Design review of the part built by this model. Coordinates are the model's own, in mm. Face numbers are marked on the shaded views. A direction names the side the tool comes from. Give positions to 0.01 mm unless a question says otherwise; leave off trailing zeros. Order: outer loops, then holes, each group sorted by start corner. A loop starts at its lowest first (then second) coordinate and runs counter-clockwise, first axis right, second up. Notation, with made-up numbers: M 80.25,77.5 L 134.25,77.5 A35 ccw 134.25,112.5 Z; hole C -29,66 d9. An arc over 180 degrees is marked long. Answer as a JSON object with one key per item and string values.
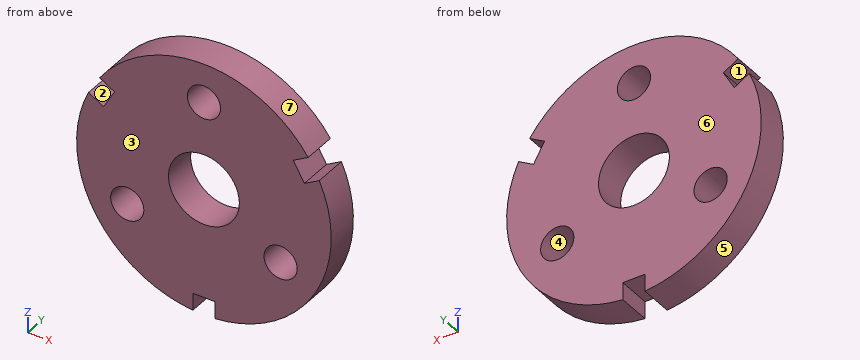
from build123d import *

# Parameters (mm, degrees)
SKETCH1_R           = 16
SKETCH1_R_2         = 7.5
BOSS_EXTRUDE1_DEPTH = 7.5


with BuildPart() as part:
    # Sketch1 → Boss-Extrude1 (new body, symmetric)
    with BuildSketch(Plane(origin=(0, 0, 0), x_dir=(1, 0, 0), z_dir=(0, 1, 0))):
        with BuildLine():
            Line((52.107837082, -24.310971075), (45.368257487, -20.419872981))
            Line((45.368257487, -20.419872981), (40.368257487, -29.080127019))
            Line((40.368257487, -29.080127019), (47.107837082, -32.971225112))
            ThreePointArc((47.107837082, -32.971225112), (0, -57.5), (-47.107837082, -32.971225112))
            Line((-47.107837082, -32.971225112), (-40.368257487, -29.080127019))
            Line((-40.368257487, -29.080127019), (-45.368257487, -20.419872981))
            Line((-45.368257487, -20.419872981), (-52.107837082, -24.310971075))
            ThreePointArc((-52.107837082, -24.310971075), (-49.796460718, 28.75), (-5, 57.282196187))
            Line((-5, 57.282196187), (-5, 49.5))
            Line((-5, 49.5), (5, 49.5))
            Line((5, 49.5), (5, 57.282196187))
            ThreePointArc((5, 57.282196187), (49.796460718, 28.75), (52.107837082, -24.310971075))
        make_face()
        Circle(SKETCH1_R, mode=Mode.SUBTRACT)
        with Locations((0, -40)):
            Circle(SKETCH1_R_2, mode=Mode.SUBTRACT)
        with Locations((-34.641016151, 20)):
            Circle(SKETCH1_R_2, mode=Mode.SUBTRACT)
        with Locations((34.641016151, 20)):
            Circle(SKETCH1_R_2, mode=Mode.SUBTRACT)
    extrude(amount=BOSS_EXTRUDE1_DEPTH, both=True)


solid = part.part
(1) We need section A-A (z = 0). Write out the cut boundary in (x, y), plus the area to 4 significant figures.
Checked values:
{"outline": "M -57.5,-7.5 L -16,-7.5 L -16,7.5 L -57.5,7.5 Z; M 16,-7.5 L 57.5,-7.5 L 57.5,7.5 L 16,7.5 Z", "area": "1,245 mm^2"}
(2) We need section C-C (z = -20). Write out the cut boundary in (x, y).
Checked values:
{"outline": "M -53.91,-7.5 L -42.14,-7.5 L -42.14,7.5 L -53.91,7.5 Z; M -27.14,-7.5 L 27.14,-7.5 L 27.14,7.5 L -27.14,7.5 Z; M 42.14,-7.5 L 53.91,-7.5 L 53.91,7.5 L 42.14,7.5 Z"}
(3) Draft analysis for pull direction Z (two halves, no side actions). For the marked faces 4, 5, 6 and 7, state which applies: +Z half, -Z half, draft (parallel to the pull), parting line (faces both ways), or undercut.
Checked values:
{"face 4": "undercut", "face 5": "parting line", "face 6": "draft", "face 7": "+Z half"}
(4) Tool access review of the marked faces 1, 2 and 3: name each direction out of +Z, -Z, +X, -X, +Y, -Y from which nothing blocks a thin tool from reaching the whole face with its end or side.
Checked values:
{"face 1": "-X, +Y, -Y", "face 2": "+Y, -Y", "face 3": "+Z, -Z, +X, -X, -Y"}
(5) We need section D-D (x = 29.5). Write out the cut boundary in (y, z).
Checked values:
{"outline": "M -7.5,-49.36 L 7.5,-49.36 L 7.5,-25.46 L -7.5,-25.46 Z; M -7.5,-14.54 L 7.5,-14.54 L 7.5,49.36 L -7.5,49.36 Z"}
(6) To check wall thickness, follow L1, parallel to Z at x = 0, y = -2.5; L2, parallel to X at y = -1, z = 0; L3, parallel to Z at x = -4, y = -1.75. State the ranges of each line that lie inside material, in increasing order. Write a range as from..to.
Checked values:
{"L1": "z = -49.5..-16, 16..32.5, 47.5..57.5", "L2": "x = -57.5..-16, 16..57.5", "L3": "z = -49.5..-15.49, 15.49..33.66, 46.34..57.36"}
(7) Insertion check: pin 1 (2.5 mm diameter, centred on y = -3, z = -52, fed in from -X); pin 2 (8 mm diameter, centred on y = -5.5, z = 13.5, fed in from +X); pin 3 (6 mm diameter, centred on x = 22, y = -2, fed in from -Z); pin 4 (17 mm diameter, centred on x = 34.64, z = -20, fed in from +Y). Each pin has a flat end and moves straight along its axis. Give the tip position at first contact, or say it passes through.
Checked values:
{"pin 1": "stops at x = -27.03", "pin 2": "stops at x = 56.71", "pin 3": "stops at z = -54.27", "pin 4": "stops at y = 7.5"}
(8) We need section B-B (x = 0). Write out the cut boundary in (y, z).
Checked values:
{"outline": "M -7.5,-49.5 L 7.5,-49.5 L 7.5,-16 L -7.5,-16 Z; M -7.5,16 L 7.5,16 L 7.5,32.5 L -7.5,32.5 Z; M -7.5,47.5 L 7.5,47.5 L 7.5,57.5 L -7.5,57.5 Z"}
